Model file for the job. Use its own axes, mm. Face numbers are marked on the shaded views. A direction names the side the tool comes from. Round coordinates to 2 decimals unless told otherwise and drop trailing zeros. Loops run counter-clockwise (first coordinate to the right, second up) from the corner with the lowest first, then second, coordinate; pieces in that order, holes last. Notation, with made-up numbers: (46, 79.5) - (52, 79.5) arc R33 cw to (52, 114.5) - close; hole circle Ø6 at (8, 2). An arc over 180 degrees is marked (long way). Answer as a JSON object with one key per item and string values.
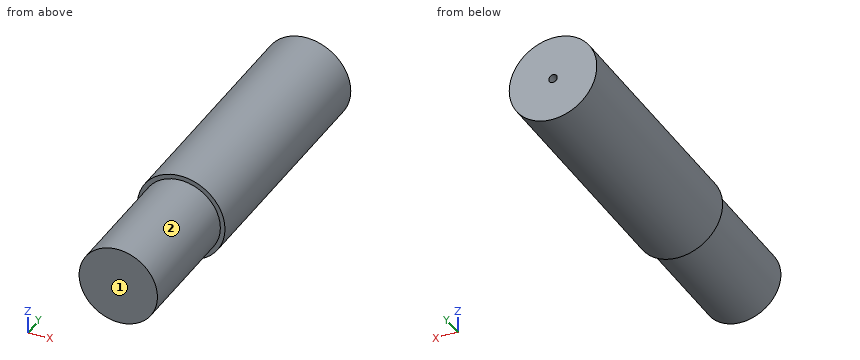
from build123d import *

# Parameters (mm, degrees)
F0_R     = 17.749636
F0_R_2   = 1.710975
F1_DEPTH = 100
F2_R     = 15.871691
F3_DEPTH = 50


with BuildPart() as f1:
    # F0 (on Front) → F1 (new body)
    with BuildSketch(Plane.XZ):
        Circle(F0_R)
        Circle(F0_R_2, mode=Mode.SUBTRACT)
    extrude(amount=-F1_DEPTH)

    # F2 (on Front) → F3 (join)
    with BuildSketch(Plane.XZ):
        Circle(F2_R)
    extrude(amount=F3_DEPTH)


solid = f1.part
1) Slice it at D-D on y = 48. List the corners of the cut face in (x, z), then the cut area to 3 significant figures.
Values follow:
{"outline": "circle Ø35.5 at (0, 0); hole circle Ø3.42 at (0, 0)", "area": "981 mm²"}
2) Slice it at A-A on z = 0. List the corners of the cut face in (x, y), then the cut area to 3 significant figures.
Values follow:
{"outline": "(-17.75, 0) - (-15.87, 0) - (-15.87, -50) - (15.87, -50) - (15.87, 0) - (17.75, 0) - (17.75, 100) - (1.71, 100) - (1.71, 0) - (-1.71, 0) - (-1.71, 100) - (-17.75, 100) - close", "area": "4,790 mm²"}
3) Drop flat-ended pins along their axis: P1, Ø1, axis at x = 10.5, y = -20.5, coming from the -Z side; P2, Ø1, axis at x = 6.5, y = -17, coming from the +Z side; P3, Ø10, axis at x = 13, y = 56.5, coming from the -Z side. Give the stop position or say it passes through.
Values follow:
{"P1": "z = -12.33", "P2": "z = 14.69", "P3": "z = -15.84"}
4) Probe probe 1 along Z at (x, y) = (0, 79); probe 2 along Y at (x, z) = (5.5, -15.5); probe 3 along Z at (x, y) = (-8, 87). List the from-to ranges inside material, lowest first.
Values follow:
{"probe 1": "-17.75 to -1.71, 1.71 to 17.75", "probe 2": "0 to 100", "probe 3": "-15.84 to 15.84"}
5) Tool access for the marked faces 1 and 2: list every direction of +Z, -Z, +X, -X, +Y, -Y with a clear straight run to the whole face (end or side of a thin tool).
Values follow:
{"face 1": "+Z, -Z, +X, -X, -Y", "face 2": "-Y"}
6) Slice it at C-C on y = -26. List the corners of the cut face in (x, z).
Values follow:
{"outline": "circle Ø31.74 at (0, 0)"}
7) Slice it at B-B on x = -11. List the corners of the cut face in (y, z), then the cut area to 3 significant figures.
Values follow:
{"outline": "(-50, -11.44) - (0, -11.44) - (0, -13.93) - (100, -13.93) - (100, 13.93) - (0, 13.93) - (0, 11.44) - (-50, 11.44) - close", "area": "3,930 mm²"}
